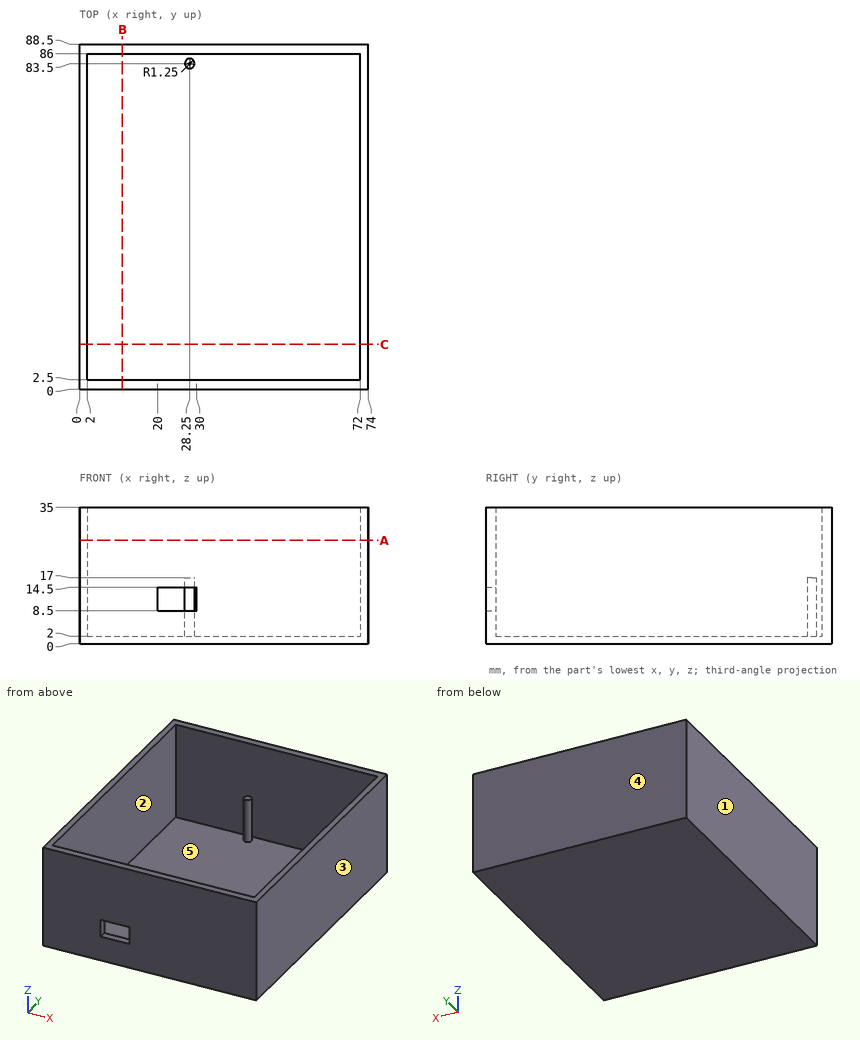
Design review of the part shown in the three views and the two pictorial views. Dimensions are in mm from the part's minimum x, y and z. A direction names the side the tool comes from. Coordinates: 2 decimals unless noted, no trailing zeros. Loops run counter-clockwise (first coordinate to the right, second up) from the corner with the lowest first, then second, coordinate; pieces in that order, holes last. Notation, with made-up numbers: M 6.5,19.25 L 62.5,19.25 A7 ccw 62.5,26.25 Z; hole C 3,23 d2. An arc over 180 degrees is marked long. One line per question, with ' | ' between items.
(1) We need section A-A (z = 26.5). Give the boundary of the cut face in (x, y), and give its area (3 significant figures).
Filled in:
outline: M 0,0 L 74,0 L 74,88.5 L 0,88.5 Z; hole M 2,2.5 L 72,2.5 L 72,86 L 2,86 Z | area: 704 mm^2
(2) We need section C-C (y = 11.5). Give the boundary of the cut face in (x, z).
Filled in:
outline: M 0,0 L 74,0 L 74,35 L 72,35 L 72,2 L 2,2 L 2,35 L 0,35 Z
(3) Draft analysis for pull direction Y (two halves, no side actions). For the marked faces 3, 4 and 5, state which applies: released by +Y, released by -Y, zero draft, split by the parting line, or undercut.
Filled in:
face 3: zero draft | face 4: released by +Y | face 5: undercut
(4) For pin 1 Ø1.2 at (x, y) = (28, 83) entering from +Z, flat-tipped, find the tip position at first contact; note if it passes through.
Filled in:
pin 1: stops at z = 17
(5) We need section B-B (x = 11). Give the boundary of the cut face in (y, z).
Filled in:
outline: M 0,0 L 88.5,0 L 88.5,35 L 86,35 L 86,2 L 2.5,2 L 2.5,35 L 0,35 Z
(6) Machinability: for the marked faces 1 and 2, which of the approach directions +Z, -Z, +X, -X, +Y, -Y give a long, thin tool a straight path to every point of the face, cutting with its end or side? Answer none if there is none.
Filled in:
face 1: +Z, -Z, -X, +Y, -Y | face 2: +Z
(7) Wall thickness on probe 1 along X at (y, z) = (16, 11); probe 2 along Y at (x, z) = (14.5, 23.5); probe 3 along Z at (x, y) = (64, 66): over which ranges is each line inside the solid? List them lowest first.
Filled in:
probe 1: x = 0 to 2, 72 to 74 | probe 2: y = 0 to 2.5, 86 to 88.5 | probe 3: z = 0 to 2
